Work out the finished part from the listing and answer in its coordinate system (mm). A direction names the side the tool comes from. Round coordinates to 2 decimals unless told otherwise and drop trailing zeros. Loops run counter-clockwise (first coordinate to the right, second up) from the corner with the lowest first, then second, coordinate; pieces in that order, holes last. Notation, with made-up numbers: (-11, 16.5) - (14, 16.5) arc R27 cw to (14, 36.5) - close; hole circle Ø2 at (8, -15.75). An arc over 180 degrees is marked (long way). Answer as CSV lines item,"result". Start each with the question number.
```python
from build123d import *

# Parameters (mm, degrees)
F1_DEPTH = 3
F2_R     = 1.185
F3_DEPTH = 3.001
F4_R     = 4.5
F5_DEPTH = 1.5
F6_R     = 2
F7_DEPTH = 4.501


with BuildPart() as f1:
    # F0 (on Top) → F1 (new body)
    with BuildSketch(Plane.XY):
        with BuildLine():
            Line((-3, 12.134661), (-9, -8.674676))
            ThreePointArc((-9, -8.674676), (0, -12.5), (9, -8.674676))
            Line((9, -8.674676), (3, 12.134661))
            ThreePointArc((3, 12.134661), (0, 12.5), (-3, 12.134661))
        make_face()
    extrude(amount=F1_DEPTH)

    # F2 (on face) → F3 (cut, through all)
    with BuildSketch(Plane.XY.offset(3)):
        with Locations((0, 9)):
            Circle(F2_R)
    extrude(amount=-F3_DEPTH, mode=Mode.SUBTRACT)

    # F4 (on face) → F5 (join)
    with BuildSketch(Plane.XY.offset(3)):
        Circle(F4_R)
    extrude(amount=F5_DEPTH)

    # F6 (on face) → F7 (cut, through all)
    with BuildSketch(Plane.XY.offset(4.5)):
        Circle(F6_R)
    extrude(amount=-F7_DEPTH, mode=Mode.SUBTRACT)


solid = f1.part
```
Item 1: Flat-ended cylindrical pins translate along their axes: pin 1 Ø2 at (x, y) = (6, -10) entering from +Z; pin 2 Ø1 at (y, z) = (-1, 2.5) entering from -X. Find the tip coordinate at first contact, or state that the pin passes through.
Item 2: Determine the mould class of faces 1 (the face through (6.042, 1.584, 1.479)), 2 (the face through (0, 12.5, 1.5)), 3 (the face through (0, -2, 2)) for opening direction X: pulls with the +X half, pulls with the -X half, needs draft (parallel to the pull), parting line crosses it, or undercut.
Item 3: Find the intervals of material crossed by L1, parallel to Y at x = 0, z = 1.1 (3 decimals); L2, parallel to Y at x = 0.5, z = 1.75; L3, parallel to Z at x = -3.25, y = 4.75, in increasing order.
Item 4: Section A-A, the plane x = 0 is taken. Give the vertices of the cut face in (y, z) (3 decimals).
Item 5: Section C-C, the plane y = 0 is taken. Give the vertices of the cut face in (x, z).
Item 6: Section D-D, the plane z = 1.8 is taken. Give the vertices of the cut face in (x, y) (3 decimals), and give its area (3 significant figures).
Item 7: Section B-B, the plane z = 3.7 is taken. Give the vertices of the cut face in (x, y), and give its area (3 significant figures).
Item 8: Which of the six approach directions +Z, -Z, +X, -X, +Y, -Y give full straight-line access (tool end or side, diameter ignored) to faces 4 (the face through (-0.1, -12.5, 1.5)), 5 (the face through (-0.59, 4.46, 3.74))?
Answer:
1,pin 1,"stops at z = 3"
1,pin 2,"stops at x = -6.93"
2,face 1,"pulls with the +X half"
2,face 2,"parting line crosses it"
2,face 3,"undercut"
3,L1,"y = -12.5 to -2, 2 to 7.815, 10.185 to 12.5"
3,L2,"y = -12.49 to -1.94, 1.94 to 7.93, 10.07 to 12.49"
3,L3,"z = 0 to 3"
4,outline,"(-12.5, 0) - (-2, 0) - (-2, 4.5) - (-4.5, 4.5) - (-4.5, 3) - (-12.5, 3) - close; (2, 0) - (7.815, 0) - (7.815, 3) - (4.5, 3) - (4.5, 4.5) - (2, 4.5) - close; (10.185, 0) - (12.5, 0) - (12.5, 3) - (10.185, 3) - close"
5,outline,"(-6.5, 0) - (-2, 0) - (-2, 4.5) - (-4.5, 4.5) - (-4.5, 3) - (-6.5, 3) - close; (2, 0) - (6.5, 0) - (6.5, 3) - (4.5, 3) - (4.5, 4.5) - (2, 4.5) - close"
6,outline,"(-9, -8.675) arc R12.5 ccw to (9, -8.675) - (3, 12.135) arc R12.5 ccw to (-3, 12.135) - close; hole circle Ø4 at (0, 0); hole circle Ø2.37 at (0, 9)"
6,area,"282 mm²"
7,outline,"circle Ø9 at (0, 0); hole circle Ø4 at (0, 0)"
7,area,"51.1 mm²"
8,face 4,"+Z, -Z, -Y"
8,face 5,"+Z"
